The listing builds one solid part. Answer for the finished solid, in the listing's coordinates (mm). A direction names the side the tool comes from. Round coordinates to 2 decimals unless told otherwise and drop trailing zeros. Order: outer loops, then holes, each group sorted by start corner. A loop starts at its lowest first (then second) coordinate and runs counter-clockwise, first axis right, second up. Notation, with made-up numbers: (38.5, 71) -> (75.5, 71) arc R19 ccw to (75.5, 83) -> close; hole circle Ø4 at (-1, 4). An arc over 180 degrees is marked (long way). Return JSON: item names as keys, results as strings. Group by question number.
(1) Each of these flat-tipped pins is pushed along its axis until it touches: pin 1 (4 mm diameter, centred on y = 616, z = 191, fed in from +X); pin 2 (1 mm diameter, centred on y = 455.5, z = 165.5, fed in from +X); pin 3 (12 mm diameter, centred on x = 26.5, y = 360.5, fed in from -Z). Where does it stop, or does it pass through?
(2) Which of the six approach directions +Z, -Z, +X, -X, +Y, -Y give full straight-line access (tool end or side, diameter ignored) to faces 5 (the face through (4, 76, 86)), 6 (the face through (19, 426, 225))?
(3) Determine the mould class of faces 1 (the face through (19.905, 426.574, 110.925)), 2 (the face through (14.99, 376.42, 115.42)), 3 (the face through (15.35, 417.02, 85.93)), 4 (the face through (0, 74, 86)) for opening direction Y: +Y half, -Y half, draft (parallel to the pull), parting line (faces both ways), or undercut.
(4) The part is cut by section C-C (z = 33.5). Determine the outline of the cut face in (x, y).
(5) The part is cut by section B-B (z = 125). Determine the outline of the cut face in (x, y).
(6) The part is cut by section A-A (y = 75). Determine the outline of the cut face in (x, z), plus the area to 3 significant figures.
(7) Consider line 1 (X direction, y = 77, z = 163); line 2 (X direction, y = 225, z = 102); line 3 (Z direction, x = 39.5, y = 794.5). Determine where each line is inside the solid, lowest interval first. Write a range as [from, to].
(8) The part is cut by section D-D (y = 599). Determine the outline of the cut face in (x, z), plus the area to 3 significant figures.
from build123d import *

# Parameters (mm, degrees)
SM_BASE_FLANGE_1_DEPTH = 225
CUT_EXTRUDE_1_DEPTH    = 10
SKETCH_7_R             = 25
CUT_EXTRUDE_2_DEPTH    = 10
SKETCH_8_R             = 25
CUT_EXTRUDE_3_DEPTH    = 10


# Sheet-metal steps are written as plain solids
with BuildPart() as part:
    # Sketch 1 → 基体-法兰1 (new body)
    with BuildSketch(Plane.XY):
        with BuildLine():
            Line((0, 0), (0, 149.77025154))
            ThreePointArc((0, 149.77025154), (0.003296983, 149.999905315), (0.013185214, 150.2293698))
            Line((0.013185214, 150.2293698), (40.172847796, 848.846293758))
            Line((40.172847796, 848.846293758), (44.166255189, 848.616734628))
            Line((44.166255189, 848.616734628), (4.006592607, 149.99981067))
            ThreePointArc((4.006592607, 149.99981067), (4.001648491, 149.885078427), (4, 149.77025154))
            Line((4, 149.77025154), (4, 0))
            Line((4, 0), (0, 0))
        make_face()
    extrude(amount=SM_BASE_FLANGE_1_DEPTH)

    # 草图6 → 切除-拉伸1 (cut)
    with BuildSketch(Plane(origin=(-8.594279324, 0.494038071, 0), x_dir=(0, 0, 1), z_dir=(-0.9983518482263736, 0.0573897825660991, 0))):
        Polygon((0, 849.752777234), (225, 849.752777234), (0, 499.752777234), align=None)
    extrude(amount=-CUT_EXTRUDE_1_DEPTH, mode=Mode.SUBTRACT)

    # 草图7 → 切除-拉伸2 (cut)
    with BuildSketch(Plane.ZY):
        with Locations((125, 75)):
            Circle(SKETCH_7_R)
    extrude(amount=-CUT_EXTRUDE_2_DEPTH, mode=Mode.SUBTRACT)

    # 草图8 → 切除-拉伸3 (cut)
    with BuildSketch(Plane(origin=(-8.594279324, 0.494038071, 0), x_dir=(0, 0, 1), z_dir=(-0.9983518482263735, 0.05738978256609909, 0))):
        with Locations(Location((125, 399.752777234, 0), (0, 0, 270))):
            Circle(SKETCH_8_R)
    extrude(amount=-CUT_EXTRUDE_3_DEPTH, mode=Mode.SUBTRACT)


solid = part.part
Answer below:
{
 "1": {"pin 1": "stops at x = 30.91", "pin 2": "stops at x = 21.6", "pin 3": "passes through"},
 "2": {"face 5": "+Z, -Z, +X, -Y", "face 6": "+Z, +X, -X, +Y, -Y"},
 "3": {"face 1": "-Y half", "face 2": "undercut", "face 3": "+Y half", "face 4": "draft"},
 "4": {"outline": "(0, 0) -> (4, 0) -> (4, 149.77) arc R4 cw to (4.01, 150) -> (27.07, 551.22) -> (23.08, 551.45) -> (0.01, 150.23) arc R8 ccw to (0, 149.77) -> close"},
 "5": {"outline": "(0, 0) -> (4, 0) -> (4, 50) -> (0, 50) -> close; (0, 100) -> (4, 100) -> (4, 149.77) arc R4 cw to (4.01, 150) -> (16.91, 374.4) -> (12.91, 374.63) -> (0.01, 150.23) arc R8 ccw to (0, 149.77) -> close; (15.78, 424.55) -> (19.78, 424.32) -> (35.24, 693.32) -> (31.25, 693.55) -> close"},
 "6": {"outline": "(0, 0) -> (4, 0) -> (4, 100) -> (0, 100) -> close; (0, 150) -> (4, 150) -> (4, 225) -> (0, 225) -> close", "area": "700 mm²"},
 "7": {"line 1": "x = [0, 4]", "line 2": "x = [4.31, 8.32]", "line 3": "z = [190.1, 225]"},
 "8": {"outline": "(25.81, 64.12) -> (29.82, 64.27) -> (29.82, 225) -> (25.81, 225) -> close", "area": "644 mm²"}
}
